The listing builds one solid part. Answer for the finished solid, in the listing's coordinates (mm). Face numbers are marked on the shaded views. A direction names the side the tool comes from. Give positions to 0.01 mm unless a question says otherwise; leave off trailing zeros. Order: outer loops, then holes, each group sorted by start corner. A loop starts at its lowest first (then second) coordinate and runs counter-clockwise, first axis right, second up. Notation, with made-up numbers: (83, 70) - (124, 70) arc R31 cw to (124, 103) - close; hole circle Ø3 at (71, 84.25). An arc over 180 degrees is marked (long way). Answer in a Markdown table with one row per item.
from build123d import *

# Parameters (mm, degrees)
CROQUIS1_R              = 4
CROQUIS1_R_2            = 1.5
CROQUIS1_R_3            = 3.5
CROQUIS1_R_4            = 1
SALIENTE_EXTRUIR1_DEPTH = 2
REDONDEO1_R             = 3
REDONDEO2_R             = 10
REDONDEO3_R             = 2
CROQUIS2_R              = 2.5
SALIENTE_EXTRUIR2_DEPTH = 5
CORTAR_EXTRUIR1_START   = -2
CROQUIS3_W              = 157.769698099
CROQUIS3_H              = 195.926743138
CORTAR_EXTRUIR1_DEPTH   = 2
CROQUIS9_W              = 5
CROQUIS9_H              = 8
SALIENTE_EXTRUIR8_DEPTH = 65
CORTAR_EXTRUIR2_DEPTH   = 5
CROQUIS11_W             = 2
CROQUIS11_H             = 3
CORTAR_EXTRUIR3_DEPTH   = 7.250462
CROQUIS12_R             = 4
CROQUIS12_R_2           = 2.5
SALIENTE_EXTRUIR9_DEPTH = 20


with BuildPart() as part:
    # Croquis1 → Saliente-Extruir1 (new body)
    with BuildSketch(Plane.XY):
        with BuildLine():
            Line((-42.426406871, 42.426406871), (-38.890872965, 45.961940777))
            Line((-38.890872965, 45.961940777), (-31.096194078, 38.16726189))
            Line((-31.096194078, 38.16726189), (-22.653119822, 29.724187634))
            ThreePointArc((-22.653119822, 29.724187634), (-19.456811617, 29.044722177), (-17.535923889, 31.688251973))
            Line((-17.535923889, 31.688251973), (-15, 80))
            Line((-15, 80), (0, 83))
            Line((0, 83), (15, 80))
            Line((15, 80), (17.535923889, 31.688251973))
            ThreePointArc((17.535923889, 31.688251973), (19.456811617, 29.044722177), (22.653119822, 29.724187634))
            Line((22.653119822, 29.724187634), (31.096194078, 38.16726189))
            Line((31.096194078, 38.16726189), (38.890872965, 45.961940777))
            Line((38.890872965, 45.961940777), (42.426406871, 42.426406871))
            Line((42.426406871, 42.426406871), (45.961940777, 38.890872965))
            Line((45.961940777, 38.890872965), (38.16726189, 31.096194078))
            Line((38.16726189, 31.096194078), (28.284271247, 21.213203436))
            ThreePointArc((28.284271247, 21.213203436), (19.497474683, 0), (28.284271247, -21.213203436))
            Line((28.284271247, -21.213203436), (38.16726189, -31.096194078))
            Line((38.16726189, -31.096194078), (45.961940777, -38.890872965))
            Line((45.961940777, -38.890872965), (42.426406871, -42.426406871))
            Line((42.426406871, -42.426406871), (38.890872965, -45.961940777))
            Line((38.890872965, -45.961940777), (31.096194078, -38.16726189))
            Line((31.096194078, -38.16726189), (22.653119822, -29.724187634))
            ThreePointArc((22.653119822, -29.724187634), (19.456811617, -29.044722177), (17.535923889, -31.688251973))
            Line((17.535923889, -31.688251973), (15, -80))
            Line((15, -80), (0, -83))
            Line((0, -83), (-15, -80))
            Line((-15, -80), (-17.535923889, -31.688251973))
            ThreePointArc((-17.535923889, -31.688251973), (-19.456811617, -29.044722177), (-22.653119822, -29.724187634))
            Line((-22.653119822, -29.724187634), (-31.096194078, -38.16726189))
            Line((-31.096194078, -38.16726189), (-38.890872965, -45.961940777))
            Line((-38.890872965, -45.961940777), (-42.426406871, -42.426406871))
            Line((-42.426406871, -42.426406871), (-45.961940777, -38.890872965))
            Line((-45.961940777, -38.890872965), (-38.16726189, -31.096194078))
            Line((-38.16726189, -31.096194078), (-28.284271247, -21.213203436))
            ThreePointArc((-28.284271247, -21.213203436), (-19.497474683, 0), (-28.284271247, 21.213203436))
            Line((-28.284271247, 21.213203436), (-38.16726189, 31.096194078))
            Line((-38.16726189, 31.096194078), (-45.961940777, 38.890872965))
            Line((-45.961940777, 38.890872965), (-42.426406871, 42.426406871))
        make_face()
        with Locations((-15.25, 15.25)):
            Circle(CROQUIS1_R, mode=Mode.SUBTRACT)
        with Locations((-24.04163056, 24.04163056)):
            Circle(CROQUIS1_R_2, mode=Mode.SUBTRACT)
        with Locations((-38.890872965, 38.890872965)):
            Circle(CROQUIS1_R_2, mode=Mode.SUBTRACT)
        with Locations(Location((38.890872965, 38.890872965, 0), (0, 0, 180))):
            Circle(CROQUIS1_R_2, mode=Mode.SUBTRACT)
        with Locations(Location((24.04163056, 24.04163056, 0), (0, 0, 180))):
            Circle(CROQUIS1_R_2, mode=Mode.SUBTRACT)
        with Locations(Location((15.25, 15.25, 0), (0, 0, 180))):
            Circle(CROQUIS1_R, mode=Mode.SUBTRACT)
        with Locations((15.25, -15.25)):
            Circle(CROQUIS1_R, mode=Mode.SUBTRACT)
        with Locations((24.04163056, -24.04163056)):
            Circle(CROQUIS1_R_2, mode=Mode.SUBTRACT)
        with Locations((38.890872965, -38.890872965)):
            Circle(CROQUIS1_R_2, mode=Mode.SUBTRACT)
        with Locations(Location((-15.25, -15.25, 0), (0, 0, 180))):
            Circle(CROQUIS1_R, mode=Mode.SUBTRACT)
        with Locations(Location((-24.04163056, -24.04163056, 0), (0, 0, 180))):
            Circle(CROQUIS1_R_2, mode=Mode.SUBTRACT)
        with Locations(Location((-38.890872965, -38.890872965, 0), (0, 0, 180))):
            Circle(CROQUIS1_R_2, mode=Mode.SUBTRACT)
        Circle(CROQUIS1_R_3, mode=Mode.SUBTRACT)
        with Locations((-11.5, -75)):
            Circle(CROQUIS1_R_2, mode=Mode.SUBTRACT)
        with Locations(Location((-14, 30, 0), (0, 0, 180))):
            Circle(CROQUIS1_R_2, mode=Mode.SUBTRACT)
        with Locations(Location((11.5, -75, 0), (0, 0, 180))):
            Circle(CROQUIS1_R_2, mode=Mode.SUBTRACT)
        with Locations((11.5, 75)):
            Circle(CROQUIS1_R_2, mode=Mode.SUBTRACT)
        with Locations(Location((-11.5, 75, 0), (0, 0, 180))):
            Circle(CROQUIS1_R_2, mode=Mode.SUBTRACT)
        with Locations((14, 30)):
            Circle(CROQUIS1_R_2, mode=Mode.SUBTRACT)
        with Locations(Location((14, -30, 0), (0, 0, 180))):
            Circle(CROQUIS1_R_2, mode=Mode.SUBTRACT)
        with Locations((-14, -30)):
            Circle(CROQUIS1_R_2, mode=Mode.SUBTRACT)
        with Locations((0, 76)):
            Circle(CROQUIS1_R_4, mode=Mode.SUBTRACT)
        with Locations(Location((0, -76, 0), (0, 0, 180))):
            Circle(CROQUIS1_R_4, mode=Mode.SUBTRACT)
        with BuildLine():
            Line((-0.620989881, -15.781703725), (-8.212878231, -22.282027547))
            ThreePointArc((-8.212878231, -22.282027547), (-8.50046857, -23.388327104), (-7.562491222, -24.04163056))
            Line((-7.562491222, -24.04163056), (8.360661842, -24.04163056))
            ThreePointArc((8.360661842, -24.04163056), (9.30628687, -23.36688939), (8.975807622, -22.253217173))
            Line((8.975807622, -22.253217173), (0.644542909, -15.75289335))
            ThreePointArc((0.644542909, -15.75289335), (0.006637615, -15.541565769), (-0.620989881, -15.781703725))
        make_face(mode=Mode.SUBTRACT)
        with BuildLine():
            Line((-7.562491222, 24.04163056), (8.360661842, 24.04163056))
            ThreePointArc((8.360661842, 24.04163056), (9.30628687, 23.36688939), (8.975807622, 22.253217173))
            Line((8.975807622, 22.253217173), (0.644542909, 15.75289335))
            ThreePointArc((0.644542909, 15.75289335), (0.006637615, 15.541565769), (-0.620989881, 15.781703725))
            Line((-0.620989881, 15.781703725), (-8.212878231, 22.282027547))
            ThreePointArc((-8.212878231, 22.282027547), (-8.50046857, 23.388327104), (-7.562491222, 24.04163056))
        make_face(mode=Mode.SUBTRACT)
        Polygon((-10, -70), (10, -70), (0, -54.625), align=None, mode=Mode.SUBTRACT)
        Polygon((0, -48.625), (-10, -33.25), (10, -33.25), align=None, mode=Mode.SUBTRACT)
        Polygon((-13.235898342, -37.299112885), (-11.768175631, -65.260618389), (-3.788893912, -51.823882197), align=None, mode=Mode.SUBTRACT)
        Polygon((3.788893912, -51.823882197), (11.768175631, -65.260618389), (13.235898342, -37.299112885), align=None, mode=Mode.SUBTRACT)
        Polygon((13.235898342, 37.299112885), (11.768175631, 65.260618389), (3.788893912, 51.823882197), align=None, mode=Mode.SUBTRACT)
        Polygon((-3.788893912, 51.823882197), (-11.768175631, 65.260618389), (-13.235898342, 37.299112885), align=None, mode=Mode.SUBTRACT)
        Polygon((-10, 33.25), (10, 33.25), (0, 48.625), align=None, mode=Mode.SUBTRACT)
        Polygon((0, 54.625), (-10, 70), (10, 70), align=None, mode=Mode.SUBTRACT)
    extrude(amount=SALIENTE_EXTRUIR1_DEPTH)

    # Redondeo1
    redondeo1_edges = [part.edges().sort_by_distance(p)[0] for p in [
        (-38.890872965, 45.961940777, 1),
        (-15, 80, 1),
        (15, 80, 1),
        (38.890872965, 45.961940777, 1),
        (45.961940777, 38.890872965, 1),
        (45.961940777, -38.890872965, 1),
        (38.890872965, -45.961940777, 1),
        (15, -80, 1),
        (-15, -80, 1),
        (-38.890872965, -45.961940777, 1),
        (-45.961940777, -38.890872965, 1),
        (-45.961940777, 38.890872965, 1),
    ]]
    fillet(redondeo1_edges, radius=REDONDEO1_R)

    # Redondeo2
    redondeo2_edges = [part.edges().sort_by_distance(p)[0] for p in [
        (0, 83, 1),
        (0, -83, 1),
    ]]
    fillet(redondeo2_edges, radius=REDONDEO2_R)

    # Redondeo3
    redondeo3_edges = [part.edges().sort_by_distance(p)[0] for p in [
        (0, -54.625, 1),
        (-10, -70, 1),
        (10, -70, 1),
        (0, -48.625, 1),
        (10, -33.25, 1),
        (-10, -33.25, 1),
        (-3.788893912, -51.823882197, 1),
        (-13.235898342, -37.299112885, 1),
        (-11.768175631, -65.260618389, 1),
        (13.235898342, -37.299112885, 1),
        (3.788893912, -51.823882197, 1),
        (11.768175631, -65.260618389, 1),
        (3.788893912, 51.823882197, 1),
        (13.235898342, 37.299112885, 1),
        (11.768175631, 65.260618389, 1),
        (-13.235898342, 37.299112885, 1),
        (-3.788893912, 51.823882197, 1),
        (-11.768175631, 65.260618389, 1),
        (0, 48.625, 1),
        (-10, 33.25, 1),
        (10, 33.25, 1),
        (0, 54.625, 1),
        (10, 70, 1),
        (-10, 70, 1),
    ]]
    fillet(redondeo3_edges, radius=REDONDEO3_R)

    # Croquis2 → Saliente-Extruir2 (add)
    with BuildSketch(Plane.XY.offset(2)):
        with BuildLine():
            Line((14, 34), (-14, 34))
            Line((-14, 34), (-24, 34))
            Line((-24, 34), (-24, 26))
            Line((-24, 26), (-14, 26))
            Line((-14, 26), (14, 26))
            ThreePointArc((14, 26), (18, 30), (14, 34))
        make_face()
        with Locations((-14, 30)):
            Circle(CROQUIS2_R, mode=Mode.SUBTRACT)
        with Locations(Location((14, 30, 0), (0, 0, 180))):
            Circle(CROQUIS2_R, mode=Mode.SUBTRACT)
    extrude(amount=SALIENTE_EXTRUIR2_DEPTH)

    # Croquis3 → Cortar-Extruir1 (cut)
    with BuildSketch(Plane.XY.offset(2).offset(CORTAR_EXTRUIR1_START)):
        with Locations((-2.348052334, 2.181833492)):
            Rectangle(CROQUIS3_W, CROQUIS3_H)
    extrude(amount=CORTAR_EXTRUIR1_DEPTH, mode=Mode.SUBTRACT)

    # Croquis9 → Saliente-Extruir8 (add, along a direction that is not the sketch's normal)
    with BuildSketch(Plane.XY.offset(7)):
        with Locations((-21.5, 30)):
            Rectangle(CROQUIS9_W, CROQUIS9_H)
    extrude(amount=SALIENTE_EXTRUIR8_DEPTH, dir=(0, -0.4226182617406976, 0.9063077870366508))

    # Croquis10 → Cortar-Extruir2 (cut)
    with BuildSketch(Plane.ZY.offset(24)):
        Polygon((65.910006157, 6.529812987), (62.845828385, -0.041337452), (65.910006157, -1.470187013), align=None)
    extrude(amount=-CORTAR_EXTRUIR2_DEPTH, mode=Mode.SUBTRACT)

    # Croquis11 → Cortar-Extruir3 (cut)
    with BuildSketch(Plane(origin=(0, 24.037394477, 11.208821127), x_dir=(1, 0, 0), z_dir=(0, -0.9063077870366509, -0.4226182617406975))):
        with Locations((-21.5, 46.47513361)):
            Rectangle(CROQUIS11_W, CROQUIS11_H)
    extrude(amount=-CORTAR_EXTRUIR3_DEPTH, mode=Mode.SUBTRACT)

    # Croquis12 → Saliente-Extruir9 (add)
    with BuildSketch(Plane.XY.offset(7)):
        with Locations(Location((-14, 30, 0), (0, 0, 270))):
            Circle(CROQUIS12_R)
        with Locations((-14, 30)):
            Circle(CROQUIS12_R_2, mode=Mode.SUBTRACT)
    extrude(amount=SALIENTE_EXTRUIR9_DEPTH)


solid = part.part
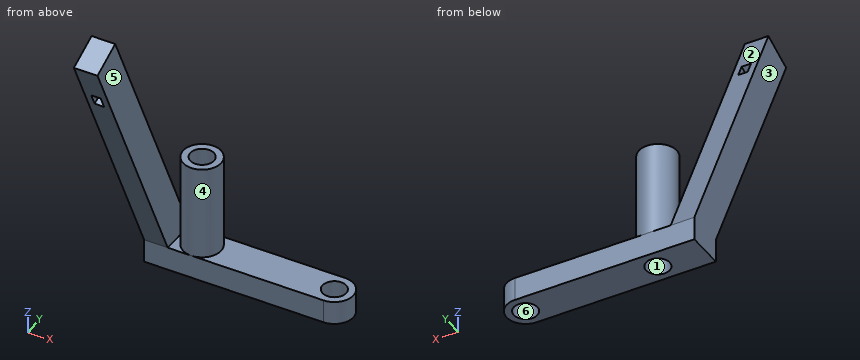
Item 1: Each of these flat-tipped pins is pushed along its axis until it touches: P1, Ø1.7, axis at y = 8.5, z = 56, coming from the +X side; P2, Ø1.5, axis at x = -3.5, y = 30, coming from the +Z side; P3, Ø1.5, axis at x = -16.5, y = 12, coming from the -Z side; P4, Ø2.5, axis at x = -14, z = 4, coming from the -Y side. Where does it stop, or does it pass through?
Answer block:
| item | result |
|---|---|
| P1 | x = -19 |
| P2 | z = 7 |
| P3 | through |
| P4 | y = 26 |
Item 2: Find section D-D on z = 35. Write down the section's boundary in (x, y), then the cut area to 3 significant figures.
Answer block:
| item | result |
|---|---|
| outline | (-24, 12.94) - (-19, 12.94) - (-19, 20.94) - (-24, 20.94) - close |
| area | 40.0 mm² |
Item 3: Consider line 1 (Y direction, x = 14, z = 4.65); line 2 (X direction, y = 30.5, z = 8); line 3 (X direction, y = 31, z = 21). Determine where each line is inside the solid, lowest interval first.
Answer block:
| item | result |
|---|---|
| line 1 | 26 to 27.5, 32.5 to 34 |
| line 2 | -24 to -19, -17.97 to -16.45, -11.55 to -10.03 |
| line 3 | -17.87 to -16.29, -11.71 to -10.13 |
Item 4: Find section B-B on y = 29. Write down the section's boundary in (x, z), then the cut area to 3 significant figures.
Answer block:
| item | result |
|---|---|
| outline | (-24, 2) - (-16.29, 2) - (-16.29, 27) - (-17.87, 27) - (-17.87, 7) - (-19, 7) - (-19, 17.72) - (-24, 17.72) - close; (-11.71, 2) - (11.71, 2) - (11.71, 7) - (-10.13, 7) - (-10.13, 27) - (-11.71, 27) - close; (16.29, 2) - (17.87, 2) - (17.87, 7) - (16.29, 7) - close |
| area | 280 mm² |
Item 5: Find section C-C on x = -5. Write down the section's boundary in (y, z), then the cut area to 3 significant figures.
Answer block:
| item | result |
|---|---|
| outline | (26, 2) - (34, 2) - (34, 7) - (26, 7) - close |
| area | 40.0 mm² |
Item 6: Which of the six approach directions +Z, -Z, +X, -X, +Y, -Y give full straight-line access (tool end or side, diameter ignored) to the marked faces 5 and 6?
Answer block:
| item | result |
|---|---|
| face 5 | +Z, +Y, -Y |
| face 6 | +Z, -Z |
Item 7: Determine the mould class of the marked faces 1, 2, 3 and 4 for opening direction X: pulls with the +X half, pulls with the -X half, needs draft (parallel to the pull), parting line crosses it, or undercut.
Answer block:
| item | result |
|---|---|
| face 1 | undercut |
| face 2 | needs draft |
| face 3 | pulls with the -X half |
| face 4 | undercut |
Item 8: Find section A-A on z = 16.5. Write down the section's boundary in (x, y).
Answer block:
| item | result |
|---|---|
| outline | (-24, 21.57) - (-19, 21.57) - (-19, 29.57) - (-24, 29.57) - close; circle Ø8 at (-14, 30); hole circle Ø5 at (-14, 30) |
